from build123d import *

# Parameters (mm, degrees)
F0_W     = 101.6
F0_H     = 44.45
F1_DEPTH = 63.5
F3_DEPTH = 127.001
F5_DEPTH = 127.001
F6_R     = 2.54
F8_DEPTH = 6.35
F9_R     = 5.08


# Not quite as in the source:
# - a pattern or mirror of a feature is missing from the dataset's text; its kind, count and spacing are read off the source's solid


with BuildPart() as f1:
    # F0 (on Front) → F1 (new body, symmetric)
    with BuildSketch(Plane.XZ):
        Rectangle(F0_W, F0_H)
    extrude(amount=F1_DEPTH, both=True)

    # F2 (on face) → F3 (cut, through all)
    with BuildSketch(Plane.XZ.offset(63.5)):
        Polygon((-50.8, -15.875), (-12.7, -15.875), (-12.7, -3.175), (-31.75, 22.225), (-50.8, 22.225), align=None)
    f3 = extrude(amount=-F3_DEPTH, mode=Mode.SUBTRACT)

    # F3_copies: F3 across plane
    add(f3.mirror(Plane(origin=(0, 0, 0), x_dir=(0, 0, 1), z_dir=(1, 0, 0))), mode=Mode.SUBTRACT)

    # F4 (on face) → F5 (cut, through all)
    with BuildSketch(Plane.XZ.offset(63.5)):
        Polygon((24.511, 22.225), (-24.511, 22.225), (-5.461, -3.175), (-5.461, -10.8996083293), (0, -13.4461144505), (5.461, -10.8996083293), (5.461, -3.175), align=None)
    extrude(amount=-F5_DEPTH, mode=Mode.SUBTRACT)

    # F6
    f6_edges = [f1.edges().sort_by_distance(p)[0] for p in [
        (-31.75, 0, 22.225),
        (-24.511, 0, 22.225),
        (24.511, 0, 22.225),
        (31.75, 0, 22.225),
    ]]
    fillet(f6_edges, radius=F6_R)

    # F7 (on face) → F8 (cut, through all)
    with BuildSketch(Plane(origin=(0, 0, -22.225), x_dir=(1, 0, 0), z_dir=(0, 0, -1))):
        with BuildLine():
            Line((-25.4, 45.72), (-50.8, 45.72))
            Line((-50.8, 45.72), (-50.8, 38.1))
            Line((-50.8, 38.1), (-25.4, 38.1))
            ThreePointArc((-25.4, 38.1), (-21.59, 41.91), (-25.4, 45.72))
        make_face()
        with BuildLine():
            Line((-25.4, -38.1), (-50.8, -38.1))
            Line((-50.8, -38.1), (-50.8, -45.72))
            Line((-50.8, -45.72), (-25.4, -45.72))
            ThreePointArc((-25.4, -45.72), (-21.59, -41.91), (-25.4, -38.1))
        make_face()
    f8 = extrude(amount=-F8_DEPTH, mode=Mode.SUBTRACT)

    # F8_copies: F8 across plane
    add(f8.mirror(Plane(origin=(0, 0, 0), x_dir=(0, 0, 1), z_dir=(1, 0, 0))), mode=Mode.SUBTRACT)

    # F9
    f9_edges = [f1.edges().sort_by_distance(p)[0] for p in [
        (-50.8, -63.5, -19.05),
        (-50.8, 63.5, -19.05),
        (50.8, -63.5, -19.05),
        (50.8, 63.5, -19.05),
        (-50.8, -45.72, -19.05),
        (-50.8, 38.1, -19.05),
        (-50.8, 45.72, -19.05),
        (-50.8, -38.1, -19.05),
        (50.8, 45.72, -19.05),
        (50.8, -45.72, -19.05),
        (50.8, -38.1, -19.05),
        (50.8, 38.1, -19.05),
    ]]
    fillet(f9_edges, radius=F9_R)


solid = f1.part
Can you work these out from the model? Positions are in its coordinate system, mm. A direction names the side the tool comes from. Round coordinates to 2 decimals unless told otherwise and drop trailing zeros. Write each loop counter-clockwise with the first axis right and the second up, starting at its lowest first coordinate (ties: lowest second). Pieces come first, ordered by that corner, then holes. Notation, with made-up numbers: (54, 41.5) -> (63, 41.5) arc R7 cw to (63, 52.5) -> close; hole circle Ø9 at (63.25, 59.25). An arc over 180 degrees is marked (long way). One line per question, with ' | ' between items. Start each with the question number.
1) Suppose I cut it at D-D on y = 41.91. Write out the boundary of the cut face in (x, z) (3 decimals).
2) Suppose I cut it at B-B on z = -9. Write out the boundary of the cut face in (x, y).
3) On a 3-axis mill with a long thin cutter (end or side, diameter ignored), from which of +Z, -Z, +X, -X, +Y, -Y can I reach the whole of each face in a straight line? I mean faces 4 (the flat face through (-20.589, -0.889, 7.344)), 5 (the flat face through (36, 45.72, -19)), 6 (the flat face through (-5.461, -1, -7)), 7 (the cylindrical face through (-21.59, -41.83, -19.09)). Say none if no direction works.
4) I'm going to push flat-ended pins straight in: P1, Ø4, axis at x = -16.5, y = 13, coming from the +Z side; P2, Ø2, axis at y = -45, z = 16.5, coming from the -X side; P3, Ø6.5, axis at y = -7.5, z = -9.5, coming from the -X side. Where does each tip first touch, or does it pass through?
5) Suppose I cut it at C-C on y = 17. Write out the boundary of the cut face in (x, z) (3 decimals).
6) Suppose I cut it at A-A on x = -38. Write out the boundary of the cut face in (y, z) (3 decimals), then the cut area to 3 significant figures.
7) If we mould it in two halves opening along X, with no side actions, what happens to faces 1 (the flat face through (-2.769, -0.889, -12.155)), 2 (the cylindrical face through (-49.351, -36.572, -19.006)), 3 (the flat face through (36, -38.1, -19))? For each: released by +X, released by -X, zero draft, split by the parting line, or undercut.
8) I need wall thicknesses on line 1 (X direction, y = -42.5, z = -3.5); line 2 (Z direction, x = -43.5, y = -16) (3 decimals); line 3 (X direction, y = -16.5, z = -3). Which ranges of each line are inside material? Lowest first, please. Write a range as [from, to].
Return value:
1) outline: (-28.702, 18.161) -> (-12.7, -3.175) -> (-12.7, -15.875) -> (-21.59, -15.875) -> (-21.59, -22.225) -> (21.59, -22.225) -> (21.59, -15.875) -> (12.7, -15.875) -> (12.7, -3.175) -> (28.702, 18.161) arc R2.54 ccw to (26.67, 22.225) -> (25.781, 22.225) arc R2.54 ccw to (23.749, 21.209) -> (5.461, -3.175) -> (5.461, -10.9) -> (0, -13.446) -> (-5.461, -10.9) -> (-5.461, -3.175) -> (-23.749, 21.209) arc R2.54 ccw to (-25.781, 22.225) -> (-26.67, 22.225) arc R2.54 ccw to start
2) outline: (-12.7, -63.5) -> (-5.46, -63.5) -> (-5.46, 63.5) -> (-12.7, 63.5) -> close; (5.46, -63.5) -> (12.7, -63.5) -> (12.7, 63.5) -> (5.46, 63.5) -> close
3) face 4: -X, +Y, -Y | face 5: -Z, +X | face 6: +Z, +Y, -Y | face 7: -Z, -X
4) P1: stops at z = 14.21 | P2: stops at x = -28.21 | P3: stops at x = -12.7
5) outline: (-50.8, -22.225) -> (50.8, -22.225) -> (50.8, -15.875) -> (12.7, -15.875) -> (12.7, -3.175) -> (28.702, 18.161) arc R2.54 ccw to (26.67, 22.225) -> (25.781, 22.225) arc R2.54 ccw to (23.749, 21.209) -> (5.461, -3.175) -> (5.461, -10.9) -> (0, -13.446) -> (-5.461, -10.9) -> (-5.461, -3.175) -> (-23.749, 21.209) arc R2.54 ccw to (-25.781, 22.225) -> (-26.67, 22.225) arc R2.54 ccw to (-28.702, 18.161) -> (-12.7, -3.175) -> (-12.7, -15.875) -> (-50.8, -15.875) -> close
6) outline: (-63.5, -22.225) -> (-45.72, -22.225) -> (-45.72, -15.875) -> (-63.5, -15.875) -> close; (-38.1, -22.225) -> (38.1, -22.225) -> (38.1, -15.875) -> (-38.1, -15.875) -> close; (45.72, -22.225) -> (63.5, -22.225) -> (63.5, -15.875) -> (45.72, -15.875) -> close | area: 710 mm2
7) face 1: undercut | face 2: released by -X | face 3: zero draft
8) line 1: x = [-12.7, -5.46], [5.46, 12.7] | line 2: z = [-22.225, -15.875] | line 3: x = [-12.83, -5.59], [5.59, 12.83]
